Geometry check sheet. Reference: the model listing, model coordinates, mm. Coordinates: 2 decimals unless noted, no trailing zeros. Answer in a Markdown table with one row per item. Add a question column.
Q1. Thickness scan on line 1 (X direction, y = 7.5, z = 0.25); line 2 (Y direction, x = 95, z = 1); line 3 (Y direction, x = 93, z = 2.1). Record the ranges inside material, lowest first.
Q2. Section check A-A, the plane y = 7. Count the separate pieces of the cut face and the enclosed holes in it, and give its area (3 significant figures).
Q3. Gauge pin test, flat ends, axial feed: P1, Ø7.5, axis at x = 95, y = 7, coming from the -Z side; P2, Ø1, axis at x = 85, z = 0.5, coming from the -Y side. Record the tip position at first contact, or that the pin passes through.
Q4. Release check for a two-part mould opening along X. For faces 1 (the face through (99.483, 8.412, 1.479)), 2 (the face through (47.7, 14.3, 3)), 3 (the face through (1.68, 3.76, 1.48)) record: pulls with the +X half, pulls with the -X half, needs draft (parallel to the pull), parting line crosses it, or undercut.
```python
from build123d import *

# Parameters (mm, degrees)
SKETCH_1_R      = 3.65
SKETCH_1_R_2    = 4.7
EXTRUDE_3_DEPTH = 3


with BuildPart() as part:
    # 草图1 → 凸台-拉伸3 (new body)
    with BuildSketch(Plane.XY):
        with BuildLine():
            ThreePointArc((90.926795434, 1.307109296), (101.665216985, 4.861102495), (95, 14))
            add(Edge.make_bspline(
                [(95, 14), (47.345961789, 28.498417982), (0, 13)],
                knots=[0.500810725, 0.500810725, 0.500810725, 1.500810725, 1.500810725, 1.500810725], degree=2))
            ThreePointArc((0, 13), (-5.732365711, 5.228000182), (3.385916999, 2.046661118))
            add(Edge.make_bspline(
                [(3.385916999, 2.046661118), (47.399803665, 26.327498122), (90.926795434, 1.307109296)],
                knots=[0, 0, 0, 1, 1, 1], degree=2))
        make_face()
        with Locations((0, 7)):
            Circle(SKETCH_1_R, mode=Mode.SUBTRACT)
        with Locations((95, 7)):
            Circle(SKETCH_1_R_2, mode=Mode.SUBTRACT)
    extrude(amount=EXTRUDE_3_DEPTH)


solid = part.part
```
Calculated:
| question | item | result |
|---|---|---|
| 1 | line 1 | x = -5.98 to -3.62, 3.62 to 14.76, 78.36 to 90.33, 99.67 to 101.98 |
| 1 | line 2 | y = 0 to 2.3, 11.7 to 14 |
| 1 | line 3 | y = 0.29 to 2.75, 11.25 to 14.6 |
| 2 | separate pieces | 4 |
| 2 | enclosed holes | 0 |
| 2 | area | 75.9 mm² |
| 3 | P1 | passes through |
| 3 | P2 | stops at y = 4.23 |
| 4 | face 1 | undercut |
| 4 | face 2 | needs draft |
| 4 | face 3 | undercut |
